Study the drawing (mm; zero at the part's minimum x, y, z) and answer. Round coordinates to 2 decimals unless told otherwise and drop trailing zeros. Order: outer loops, then holes, each group sorted by start corner. A loop starts at its lowest first (then second) coordinate and runs counter-clockwise, first axis right, second up. Notation, with made-up numbers: (14, -40) -> (35, -40) arc R28 ccw to (35, -3) -> close; hole circle Ø7 at (-22, 2). An arc over 180 degrees is marked (long way). Use one line per item in the form item = value.
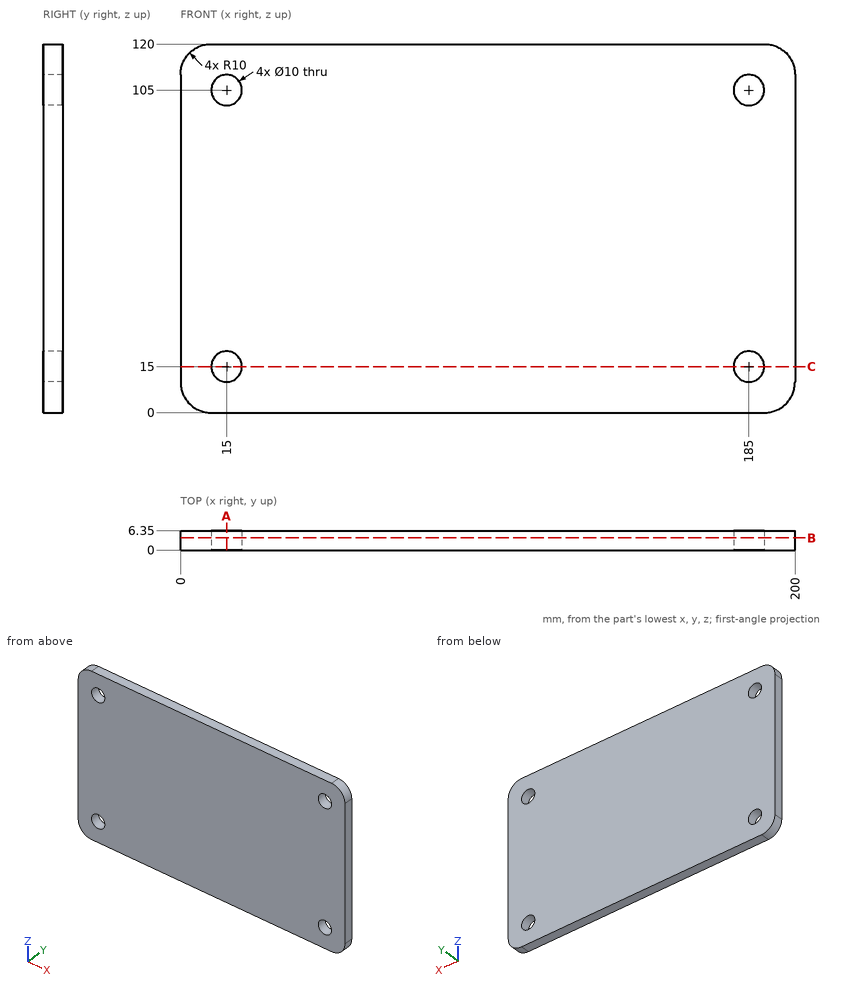
Item 1: The part is cut by section B-B, the plane y = 4. Give the vertices of the cut face in (x, z), and give its area (3 significant figures).
Findings:
outline = (0, 10) arc R10 ccw to (10, 0) -> (190, 0) arc R10 ccw to (200, 10) -> (200, 110) arc R10 ccw to (190, 120) -> (10, 120) arc R10 ccw to (0, 110) -> close; hole circle Ø10 at (15, 15); hole circle Ø10 at (15, 105); hole circle Ø10 at (185, 15); hole circle Ø10 at (185, 105)
area = 23,600 mm^2
Item 2: The part is cut by section A-A, the plane x = 15. Give the vertices of the cut face in (y, z), and give its area (3 significant figures).
Findings:
outline = (0, 0) -> (6.35, 0) -> (6.35, 10) -> (0, 10) -> close; (0, 20) -> (6.35, 20) -> (6.35, 100) -> (0, 100) -> close; (0, 110) -> (6.35, 110) -> (6.35, 120) -> (0, 120) -> close
area = 635 mm^2
Item 3: Consider line 1 along X through (y, z) = (2.75, 105); line 2 along Z through (x, y) = (185, 3.75); line 3 along X through (y, z) = (5.5, 108). Determine where each line is inside the solid, lowest interval first.
Findings:
line_1 = 0 to 10, 20 to 180, 190 to 200
line_2 = 0 to 10, 20 to 100, 110 to 120
line_3 = 0 to 11, 19 to 181, 189 to 200
Item 4: The part is cut by section C-C, the plane z = 15. Give the vertices of the cut face in (x, y), and give its area (3 significant figures).
Findings:
outline = (0, 0) -> (10, 0) -> (10, 6.35) -> (0, 6.35) -> close; (20, 0) -> (180, 0) -> (180, 6.35) -> (20, 6.35) -> close; (190, 0) -> (200, 0) -> (200, 6.35) -> (190, 6.35) -> close
area = 1,140 mm^2
